```python
from build123d import *

# Parameters (mm, degrees)
SKETCH1_W           = 101.6
SKETCH1_H           = 203.2
BOSS_EXTRUDE1_DEPTH = 50.8
SHELL1_T            = 2.54
SKETCH2_R           = 1.5875
CUT_EXTRUDE1_DEPTH  = 50.8
BOSS_EXTRUDE2_REACH = 130.59
SKETCH3_R           = 3.592102448
SKETCH4_R           = 1.5875
CUT_EXTRUDE2_DEPTH  = 130.880848574
CUT_EXTRUDE3_DEPTH  = 159.909484662


with BuildPart() as part:
    # Sketch1 → Boss-Extrude1 (new body)
    with BuildSketch(Plane.XY):
        Rectangle(SKETCH1_W, SKETCH1_H)
    extrude(amount=BOSS_EXTRUDE1_DEPTH)

    # Shell1
    shell1_openings = [part.faces().sort_by_distance(p)[0] for p in [
        (0, 0, 50.8),
    ]]
    offset(amount=SHELL1_T, openings=shell1_openings, kind=Kind.INTERSECTION)

    # Sketch2 → Cut-Extrude1 (cut)
    with BuildSketch(Plane.XY):
        with Locations((0, 31.018508685)):
            Circle(SKETCH2_R)
        with Locations((0, -31.018508685)):
            Circle(SKETCH2_R)
    extrude(amount=-CUT_EXTRUDE1_DEPTH, mode=Mode.SUBTRACT)

    # Boss-Extrude2: up to this face of the body (flat: up to its plane)
    boss_extrude2_end = Plane(part.part.faces().sort_by_distance((0, 0, -2.54))[0])
    # Sketch3 → Boss-Extrude2 (add, up to the picked face)
    with BuildSketch(Plane.XY.offset(50.8), mode=Mode.PRIVATE) as boss_extrude2_sk1:
        with Locations((-50.8, 101.6)):
            Circle(SKETCH3_R)
    boss_extrude2_tool1 = split(extrude(boss_extrude2_sk1.sketch, amount=-BOSS_EXTRUDE2_REACH, mode=Mode.PRIVATE), bisect_by=boss_extrude2_end, keep=Keep.BOTH, mode=Mode.PRIVATE)
    # Sketch3 → Boss-Extrude2 (add, up to the picked face)
    with BuildSketch(Plane.XY.offset(50.8), mode=Mode.PRIVATE) as boss_extrude2_sk2:
        with Locations((50.8, 101.6)):
            Circle(SKETCH3_R)
    boss_extrude2_tool2 = split(extrude(boss_extrude2_sk2.sketch, amount=-BOSS_EXTRUDE2_REACH, mode=Mode.PRIVATE), bisect_by=boss_extrude2_end, keep=Keep.BOTH, mode=Mode.PRIVATE)
    # Sketch3 → Boss-Extrude2 (add, up to the picked face)
    with BuildSketch(Plane.XY.offset(50.8), mode=Mode.PRIVATE) as boss_extrude2_sk3:
        with Locations((50.8, -101.6)):
            Circle(SKETCH3_R)
    boss_extrude2_tool3 = split(extrude(boss_extrude2_sk3.sketch, amount=-BOSS_EXTRUDE2_REACH, mode=Mode.PRIVATE), bisect_by=boss_extrude2_end, keep=Keep.BOTH, mode=Mode.PRIVATE)
    # Sketch3 → Boss-Extrude2 (add, up to the picked face)
    with BuildSketch(Plane.XY.offset(50.8), mode=Mode.PRIVATE) as boss_extrude2_sk4:
        with Locations((-50.8, -101.6)):
            Circle(SKETCH3_R)
    boss_extrude2_tool4 = split(extrude(boss_extrude2_sk4.sketch, amount=-BOSS_EXTRUDE2_REACH, mode=Mode.PRIVATE), bisect_by=boss_extrude2_end, keep=Keep.BOTH, mode=Mode.PRIVATE)
    # Sketch3 → Boss-Extrude2 (add, up to the picked face)
    with BuildSketch(Plane.XY.offset(50.8), mode=Mode.PRIVATE) as boss_extrude2_sk5:
        with Locations((-50.8, 0)):
            Circle(SKETCH3_R)
    boss_extrude2_tool5 = split(extrude(boss_extrude2_sk5.sketch, amount=-BOSS_EXTRUDE2_REACH, mode=Mode.PRIVATE), bisect_by=boss_extrude2_end, keep=Keep.BOTH, mode=Mode.PRIVATE)
    # Sketch3 → Boss-Extrude2 (add, up to the picked face)
    with BuildSketch(Plane.XY.offset(50.8), mode=Mode.PRIVATE) as boss_extrude2_sk6:
        with Locations((50.8, 0)):
            Circle(SKETCH3_R)
    boss_extrude2_tool6 = split(extrude(boss_extrude2_sk6.sketch, amount=-BOSS_EXTRUDE2_REACH, mode=Mode.PRIVATE), bisect_by=boss_extrude2_end, keep=Keep.BOTH, mode=Mode.PRIVATE)
    add(boss_extrude2_tool1.solids().sort_by(Axis((-50.8, 101.6, 50.8), (0, 0, -1)))[0])
    add(boss_extrude2_tool2.solids().sort_by(Axis((50.8, 101.6, 50.8), (0, 0, -1)))[0])
    add(boss_extrude2_tool3.solids().sort_by(Axis((50.8, -101.6, 50.8), (0, 0, -1)))[0])
    add(boss_extrude2_tool4.solids().sort_by(Axis((-50.8, -101.6, 50.8), (0, 0, -1)))[0])
    add(boss_extrude2_tool5.solids().sort_by(Axis((-50.8, 0, 50.8), (0, 0, -1)))[0])
    add(boss_extrude2_tool6.solids().sort_by(Axis((50.8, 0, 50.8), (0, 0, -1)))[0])

    # Sketch4 → Cut-Extrude2 (cut, through all)
    with BuildSketch(Plane.XY.offset(50.8)):
        with Locations((-50.8, 0)):
            Circle(SKETCH4_R)
        with Locations((50.8, 0)):
            Circle(SKETCH4_R)
        with Locations((50.8, 101.6)):
            Circle(SKETCH4_R)
        with Locations((-50.8, 101.6)):
            Circle(SKETCH4_R)
        with Locations((50.8, -101.6)):
            Circle(SKETCH4_R)
        with Locations((-50.8, -101.6)):
            Circle(SKETCH4_R)
    extrude(amount=-CUT_EXTRUDE2_DEPTH, mode=Mode.SUBTRACT)

    # Sketch5 → Cut-Extrude3 (cut, through all)
    with BuildSketch(Plane(origin=(53.34, 0, 0), x_dir=(0, 0, -1), z_dir=(1, 0, 0))):
        with BuildLine():
            Line((-17.78, 88.01360889), (-17.78, 13.58639111))
            ThreePointArc((-17.78, 13.58639111), (-24.13, 7.23639111), (-30.48, 13.58639111))
            Line((-30.48, 13.58639111), (-30.48, 88.01360889))
            ThreePointArc((-30.48, 88.01360889), (-24.13, 94.36360889), (-17.78, 88.01360889))
        make_face()
    cut_extrude3 = extrude(amount=-CUT_EXTRUDE3_DEPTH, mode=Mode.SUBTRACT)

    # Mirror1: Cut-Extrude3 across plane
    add(cut_extrude3.mirror(Plane.ZX), mode=Mode.SUBTRACT)


solid = part.part
```
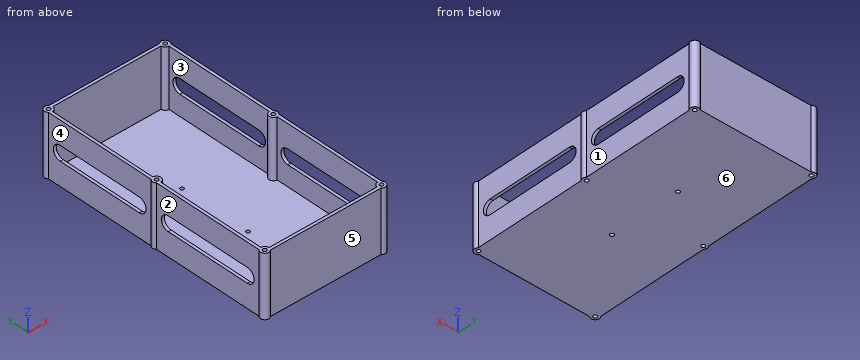
Geometry check sheet. Reference: the model listing, model coordinates, mm. Face numbers are marked on the shaded views. A direction names the side the tool comes from. Give positions to 0.01 mm unless a question says otherwise; leave off trailing zeros. Order: outer loops, then holes, each group sorted by start corner. A loop starts at its lowest first (then second) coordinate and runs counter-clockwise, first axis right, second up.
1. Section check C-C, the plane x = -10. Enter the section's corners in (y, z).
2. Access from +Z, -Z, +X, -X, +Y, -Y to the whole of each face (thin tool, end or side, straight path). Record for the marked faces 1, 2 and 3.
3. Gauge pin test, flat ends, axial feed: pin 1 Ø2 at (x, y) = (-13.5, -22.5) entering from +Z; pin 2 Ø6 at (x, z) = (-39.5, 42) entering from -Y; pin 3 Ø3 at (y, z) = (-58, 37) entering from +X. Record the tip position at first contact, or that the pin passes through.
4. Section check B-B, the plane z = 33.5. Give the number of separate pieces and of enclosed holes in the cut face, and give its area (3 significant figures).
5. Section check A-A, the plane y = 46. Enter the section's corners in (x, z), and give its area (3 significant figures).
6. Release check for a two-part mould opening along Y. For the marked faces 4, 5 and 6 record: pulls with the +Y half, pulls with the -Y half, needs draft (parallel to the pull), parting line crosses it, or undercut.
7. Thickness scan on L1, parallel to Y at x = 0, z = -2; L2, parallel to Y at x = -23.5, z = 23.5; L3, parallel to X at y = -95.5, z = 44.5. Record the ranges inside material, lowest first.
Values follow:
1. outline: (-104.14, -2.54) - (104.14, -2.54) - (104.14, 50.8) - (101.6, 50.8) - (101.6, 0) - (-101.6, 0) - (-101.6, 50.8) - (-104.14, 50.8) - close
2. face 1: +Z, -Z, +X
2. face 2: +Z, -Z, -X
2. face 3: +Z
3. pin 1: stops at z = 0
3. pin 2: stops at y = -104.14
3. pin 3: stops at x = 53.34
4. separate pieces: 1
4. enclosed holes: 7
4. area: 1,640 mm2
5. outline: (-53.34, -2.54) - (53.34, -2.54) - (53.34, 17.78) - (50.8, 17.78) - (50.8, 0) - (-50.8, 0) - (-50.8, 17.78) - (-53.34, 17.78) - close; (-53.34, 30.48) - (-50.8, 30.48) - (-50.8, 50.8) - (-53.34, 50.8) - close; (50.8, 30.48) - (53.34, 30.48) - (53.34, 50.8) - (50.8, 50.8) - close
5. area: 465 mm2
6. face 4: undercut
6. face 5: pulls with the -Y half
6. face 6: needs draft
7. L1: y = -104.14 to -32.61, -29.43 to 29.43, 32.61 to 104.14
7. L2: y = -104.14 to -101.6, 101.6 to 104.14
7. L3: x = -53.34 to -50.8, 50.8 to 53.34
